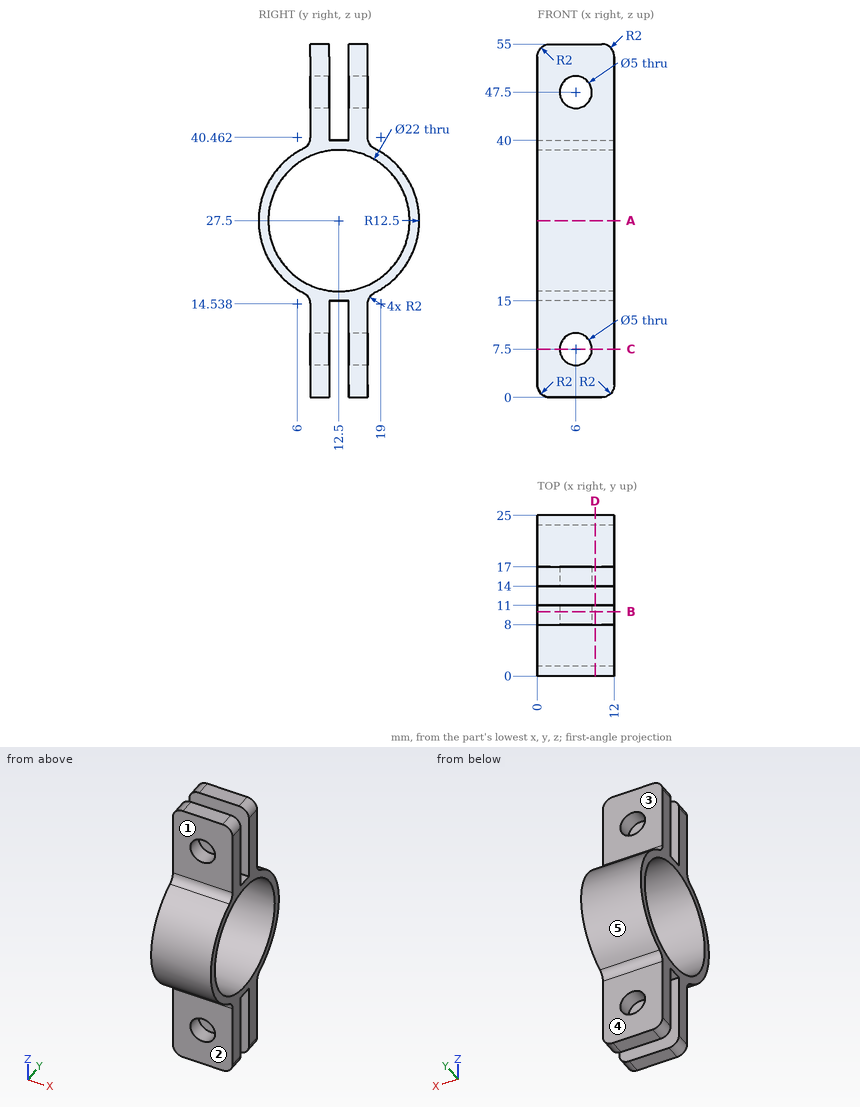
Geometry: see drawing. Coordinates: mm, zero at the bounding-box minimum. A direction names the side the tool comes from. Round coordinates to 2 decimals unless told otherwise and drop trailing zeros. Order: outer loops, then holes, each group sorted by start corner. A loop starts at its lowest first (then second) coordinate and runs counter-clockwise, first axis right, second up. Notation, with made-up numbers: (-17.5, -15.5) -> (7.5, -15.5) arc R31 cw to (7.5, 15.5) -> close; hole circle Ø11 at (37.5, 44.25). An arc over 180 degrees is marked (long way). Answer as CSV lines item,"result".
Item 1: Section B-B, the plane y = 10. Return loops of the section in (x, z).
A:
outline,"(0, 2) arc R2 ccw to (2, 0) -> (10, 0) arc R2 ccw to (12, 2) -> (12, 16.79) -> (0, 16.79) -> close; (0, 38.21) -> (12, 38.21) -> (12, 53) arc R2 ccw to (10, 55) -> (2, 55) arc R2 ccw to (0, 53) -> close; hole circle Ø5 at (6, 7.5); hole circle Ø5 at (6, 47.5)"
Item 2: Section C-C, the plane z = 7.5. Return loops of the section in (x, y).
A:
outline,"(0, 8) -> (3.5, 8) -> (3.5, 11) -> (0, 11) -> close; (0, 14) -> (3.5, 14) -> (3.5, 17) -> (0, 17) -> close; (8.5, 8) -> (12, 8) -> (12, 11) -> (8.5, 11) -> close; (8.5, 14) -> (12, 14) -> (12, 17) -> (8.5, 17) -> close"
Item 3: Pin query (flat end, axial travel): pin 1 Ø1.5 at (x, y) = (8, 12) entering from +Z; pin 2 Ø1 at (y, z) = (4.5, 16.5) entering from -X; pin 3 Ø2 at (x, y) = (10.5, 21) entering from -Z; pin 4 Ø0.9 at (x, y) = (5.5, 12.5) entering from -Z. Return the tip coordinate at first contact, or that it passes through.
A:
pin 1,"z = 40"
pin 2,"through"
pin 3,"z = 17.5"
pin 4,"z = 15"
Item 4: Line query: L1, parallel to Y at x = 11.5, z = 12.5; L2, parallel to X at y = 14.85, z = 47.5; L3, parallel to Z at x = 6, y = 9.45. Output: solid intervals per line, ascending.
A:
L1,"8 to 11, 14 to 17"
L2,"0 to 3.5, 8.5 to 12"
L3,"0 to 5, 10 to 16.93, 38.07 to 45, 50 to 55"
Item 5: Section A-A, the plane z = 27.5. Return loops of the section in (x, y).
A:
outline,"(0, 0) -> (12, 0) -> (12, 1.5) -> (0, 1.5) -> close; (0, 23.5) -> (12, 23.5) -> (12, 25) -> (0, 25) -> close"
Item 6: Reachability of the marked faces 1, 2, 3, 4 and 5 from +Z, -Z, +X, -X, +Y, -Y: full face, straight path, thin tool, end or side. Return the list, or none.
A:
face 1,"+Z, +X, -X, -Y"
face 2,"-Z, +X, -X, -Y"
face 3,"+Z, +X, -X, +Y"
face 4,"-Z, +X, -X, +Y"
face 5,"+X, -X, +Y"
Item 7: Section D-D, the plane x = 9. Return loops of the section in (y, z), plus the area to 3 significant figures.
A:
outline,"(6.9, 16.33) arc R2 cw to (8, 14.54) -> (8, 0) -> (11, 0) -> (11, 15) -> (14, 15) -> (14, 0) -> (17, 0) -> (17, 14.54) arc R2 cw to (18.1, 16.33) arc R12.5 ccw to (18.1, 38.67) arc R2 cw to (17, 40.46) -> (17, 55) -> (14, 55) -> (14, 40) -> (11, 40) -> (11, 55) -> (8, 55) -> (8, 40.46) arc R2 cw to (6.9, 38.67) arc R12.5 ccw to start; hole circle Ø22 at (12.5, 27.5)"
area,"297 mm²"
